```python
from build123d import *

# Parameters (mm, degrees)
SZKIC1_R                                     = 14
SZKIC1_R_2                                   = 10
DODANIE_WYCI_GNI_CIE1_DEPTH                  = 380
SZKIC2_W                                     = 15
SZKIC2_H                                     = 15
DODANIE_WYCI_GNI_CIE2_DEPTH                  = 12
DODANIE_WYCI_GNI_CIE2_DIRECTION_2_REACH      = 383.287
DODANIE_WYCI_GNI_CIE2_DIRECTION_2_END_RADIUS = 14
ZAOKR_GLENIE1_RADIUS                         = 7.5
ZAOKR_GLENIE1_LENGTH                         = 15
SZKIC3_R                                     = 4.5
WYTNIJ_WYCI_GNI_CIE1_DEPTH                   = 382.4947575
SFAZOWANIE2_SIZE                             = 2
ZAOKR_GLENIE2_R                              = 3


with BuildPart() as part:
    # Szkic1 → Dodanie-wyciągnięcie1 (new body)
    with BuildSketch(Plane(origin=(0, 0, 0), x_dir=(1, 0, 0), z_dir=(0, 1, 0))):
        with Locations(Location((0, 0, 0), (0, 0, 270))):
            Circle(SZKIC1_R)
        with Locations(Location((0, 0, 0), (0, 0, 270))):
            Circle(SZKIC1_R_2, mode=Mode.SUBTRACT)
    extrude(amount=DODANIE_WYCI_GNI_CIE1_DEPTH)

    # Szkic2 → Dodanie-wyciągnięcie2 (add)
    with BuildSketch(Plane.XY.offset(14)):
        with Locations((0, 12.5)):
            Rectangle(SZKIC2_W, SZKIC2_H)
    extrude(amount=DODANIE_WYCI_GNI_CIE2_DEPTH)

    # Dodanie-wyciągnięcie2 direction 2: up to this cylinder (the profile starts outside it)
    dodanie_wyci_gni_cie2_direction_2_end = Plane(origin=(0, 12.5, 0), z_dir=(0, -1, 0)) * Cylinder(DODANIE_WYCI_GNI_CIE2_DIRECTION_2_END_RADIUS, 795.574, mode=Mode.PRIVATE)
    # Szkic2 → Dodanie-wyciągnięcie2 direction 2 (add, up to the surface)
    with BuildSketch(Plane.XY.offset(14), mode=Mode.PRIVATE) as dodanie_wyci_gni_cie2_direction_2_sk1:
        with Locations((0, 12.5)):
            Rectangle(SZKIC2_W, SZKIC2_H)
    dodanie_wyci_gni_cie2_direction_2_tool1 = extrude(dodanie_wyci_gni_cie2_direction_2_sk1.sketch, amount=-DODANIE_WYCI_GNI_CIE2_DIRECTION_2_REACH, mode=Mode.PRIVATE) - dodanie_wyci_gni_cie2_direction_2_end
    add(dodanie_wyci_gni_cie2_direction_2_tool1.solids().sort_by_distance((0, 12.5, 14))[0])
    add(dodanie_wyci_gni_cie2_direction_2_tool1.solids().sort_by_distance((0, 12.5, 14))[1])

    # Zaokrąglenie1: full round fillet: the end face becomes a half cylinder, R = half its width
    zaokr_glenie1_face = Plane((0, 12.5, 26), x_dir=(1, 0, 0), z_dir=(0, 0, 1))  # on the end face: x along it, z out of the body
    zaokr_glenie1_slab = zaokr_glenie1_face.offset(-ZAOKR_GLENIE1_RADIUS / 2) * Box(ZAOKR_GLENIE1_LENGTH, 2 * ZAOKR_GLENIE1_RADIUS, ZAOKR_GLENIE1_RADIUS, mode=Mode.PRIVATE)  # the body's end, R deep
    zaokr_glenie1_round = Plane((0, 12.5, 18.5), x_dir=(0, 0, 1), z_dir=(1, 0, 0)) * Cylinder(ZAOKR_GLENIE1_RADIUS, ZAOKR_GLENIE1_LENGTH, mode=Mode.PRIVATE)  # its axis R under the face
    add(zaokr_glenie1_slab - zaokr_glenie1_round, mode=Mode.SUBTRACT)

    # Szkic3 → Wytnij-wyciągnięcie1 (cut, through all)
    with BuildSketch(Plane(origin=(7.5, 0, 0), x_dir=(0, 0, -1), z_dir=(1, 0, 0))):
        with Locations(Location((-18.5, 12.5, 0), (0, 0, 90))):
            Circle(SZKIC3_R)
    extrude(amount=-WYTNIJ_WYCI_GNI_CIE1_DEPTH, mode=Mode.SUBTRACT)

    # Sfazowanie2
    sfazowanie2_edges = [part.edges().sort_by_distance(p)[0] for p in [
        (-7.5, 8, 18.5),
        (7.5, 8, 18.5),
    ]]
    chamfer(sfazowanie2_edges, length=SFAZOWANIE2_SIZE)

    # Zaokrąglenie2
    zaokr_glenie2_edges = [part.edges().sort_by_distance(p)[0] for p in [
        (0, 0, -14),
    ]]
    fillet(zaokr_glenie2_edges, radius=ZAOKR_GLENIE2_R)


solid = part.part
```
Design review of the part built by this model. Coordinates are the model's own, in mm. A direction names the side the tool comes from. Round coordinates to 2 decimals unless told otherwise and drop trailing zeros. Write each loop counter-clockwise with the first axis right and the second up, starting at its lowest first coordinate (ties: lowest second). Pieces come first, ordered by that corner, then holes. Notation, with made-up numbers: (3.5, -32) -> (36.5, -32) arc R31 ccw to (36.5, -8) -> close; hole circle Ø9 at (25, 66). An arc over 180 degrees is marked (long way). Answer in a Markdown table with one row per item.
Q1. Clearance check with flat-ended pins moving along their axes: pin 1 Ø3 at (x, y) = (4, 286) entering from -Z (3 decimals); pin 2 Ø4 at (y, z) = (97.5, 3) entering from -X; pin 3 Ø8 at (y, z) = (137.5, 21) entering from -X; pin 4 Ø7.5 at (x, z) = (-2.5, 15) entering from -Y (3 decimals). State where each tip first meets the part, or that it passes through.
The answers:
| item | result |
|---|---|
| pin 1 | z = -13.775 |
| pin 2 | x = -13.96 |
| pin 3 | through |
| pin 4 | y = 0.035 |
Q2. For faces 1 (the face through (-10, 0, 2)), 2 (the face through (-7.5, 10, 12)), 3 (the face through (7.5, 10, 12)), list the 3-axis set-ups (+Z, -Z, +X, -X, +Y, -Y) from which the entire face can be reached by the end or side of a thin tool; tool diameter is ignored.
The answers:
| item | result |
|---|---|
| face 1 | +Z, -Z, +X, -X, -Y |
| face 2 | +Z, -X, +Y, -Y |
| face 3 | +Z, +X, +Y, -Y |
Q3. Take a section at A-A, the plane x = 0. State the section outline as (y, z) points, then the cut area to 3 significant figures.
The answers:
| item | result |
|---|---|
| outline | (0, -11) arc R3 ccw to (3, -14) -> (380, -14) -> (380, -10) -> (0, -10) -> close; (0, 10) -> (380, 10) -> (380, 14) -> (20, 14) -> (20, 18.5) arc R7.5 ccw to (5, 18.5) -> (5, 14) -> (3, 14) arc R3 ccw to (0, 11) -> close; hole circle Ø9 at (12.5, 18.5) |
| area | 3,130 mm² |
Q4. Take a section at B-B, the plane y = 12.5. State the section outline as (x, z) points, then the cut area to 3 significant figures.
The answers:
| item | result |
|---|---|
| outline | (-7.5, 11.82) arc R14 ccw (long way) to (7.5, 11.82) -> (7.5, 12) -> (5.5, 14) -> (-5.5, 14) -> (-7.5, 12) -> close; (-7.5, 25) -> (-5.5, 23) -> (5.5, 23) -> (7.5, 25) -> (7.5, 26) -> (-7.5, 26) -> close; hole circle Ø20 at (0, 0) |
| area | 349 mm² |
Q5. Take a section at D-D, the plane y = 320. State the section outline as (x, z) points.
The answers:
| item | result |
|---|---|
| outline | circle Ø28 at (0, 0); hole circle Ø20 at (0, 0) |
Q6. To check wall thickness, follow L1, parallel to Z at x = 1, y = 129; L2, parallel to X at y = 95, z = 0; L3, parallel to X at y = 282, z = -1.5. State the ranges of each line that lie inside material, in increasing order. Write a range as [from, to].
The answers:
| item | result |
|---|---|
| L1 | [-13.96, -9.95], [9.95, 13.96] |
| L2 | [-14, -10], [10, 14] |
| L3 | [-13.92, -9.89], [9.89, 13.92] |
Q7. Draft analysis for pull direction Z (two halves, no side actions). For faces 4 (the face through (0, 5, 16)), 5 (the face through (0.077, 14.919, 22.294)), 6 (the face through (0.11, 12.66, 26)), 7 (the face through (-9.76, 187.34, -2.17)), state which applies: +Z half, -Z half, draft (parallel to the pull), parting line (faces both ways), or undercut.
The answers:
| item | result |
|---|---|
| face 4 | draft |
| face 5 | undercut |
| face 6 | +Z half |
| face 7 | undercut |
Q8. Take a section at C-C, the plane z = 0. State the section outline as (x, y) points.
The answers:
| item | result |
|---|---|
| outline | (-14, 3) arc R3 ccw to (-11, 0) -> (-10, 0) -> (-10, 380) -> (-14, 380) -> close; (10, 0) -> (11, 0) arc R3 ccw to (14, 3) -> (14, 380) -> (10, 380) -> close |
